Input: part model. Units: mm. Frame: model coordinates. Coordinates: 2 decimals unless noted, no trailing zeros. Loops run counter-clockwise (first coordinate to the right, second up) from the corner with the lowest first, then second, coordinate; pieces in that order, holes last. Notation, with made-up numbers: (49.5, 89.25) - (65.5, 89.25) arc R25 ccw to (65.5, 126.25) - close; hole circle Ø7 at (14, 42). An arc over 180 degrees is marked (long way). Use one line per item in the form item = value.
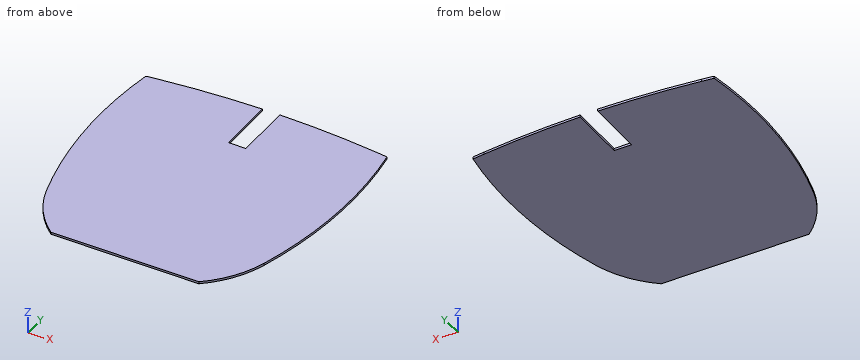
from build123d import *

# Parameters (mm, degrees)
F1_DEPTH = 0.5


with BuildPart() as f1:
    # F0 (on Top) → F1 (new body)
    with BuildSketch(Plane.XY):
        with BuildLine():
            ThreePointArc((-2, 57.790434), (-13.520553, 57.362383), (-25, 56.3))
            ThreePointArc((-25, 56.3), (-26.350558, 56.132887), (-27.7, 55.956987))
            ThreePointArc((-27.7, 55.956987), (-28.812855, 33.827216), (-25, 12))
            ThreePointArc((-25, 12), (-21.917468, 5.388354), (-17, 0))
            Line((-17, 0), (17, 0))
            ThreePointArc((17, 0), (21.917468, 5.388354), (25, 12))
            ThreePointArc((25, 12), (28.812855, 33.827216), (27.7, 55.956987))
            ThreePointArc((27.7, 55.956987), (26.350558, 56.132887), (25, 56.3))
            ThreePointArc((25, 56.3), (13.520553, 57.362383), (2, 57.790434))
            Line((2, 57.790434), (2, 44.4))
            Line((2, 44.4), (-2, 44.4))
            Line((-2, 44.4), (-2, 57.790434))
        make_face()
    extrude(amount=F1_DEPTH)


solid = f1.part
Q1. Ray query, line 1 along Y through (x, z) = (-1, 0.3); line 2 along X through (y, z) = (49, 0.15); line 3 along Y through (x, z) = (-3, 0.15). Return the intervals inside material, ascending. Write a range as [from, to].
Check values:
line_1 = [0, 44.4]
line_2 = [-28.59, -2], [2, 28.59]
line_3 = [0, 57.78]
Q2. Cut plane A-A, the plane y = 51. Return loops of the section in (x, z), then the cut area to 3 significant figures.
Check values:
outline = (-28.38, 0) - (-2, 0) - (-2, 0.5) - (-28.38, 0.5) - close; (2, 0) - (28.38, 0) - (28.38, 0.5) - (2, 0.5) - close
area = 26.4 mm²
Q3. Cut plane C-C, the plane x = -18. Return loops of the section in (y, z).
Check values:
outline = (0.85, 0) - (57.02, 0) - (57.02, 0.5) - (0.85, 0.5) - close
Q4. First-contact query: P1, Ø10, axis at x = 20.5, y = 20, coming from the -Z side. Flat tip, straight axial feed; report the tip coordinate or a pass-through.
Check values:
P1 = 0
Q5. Cut plane D-D, the plane y = 4. Return loops of the section in (x, z), then the cut area to 3 significant figures.
Check values:
outline = (-20.92, 0) - (20.92, 0) - (20.92, 0.5) - (-20.92, 0.5) - close
area = 20.9 mm²
Q6. Cut plane B-B, the plane z = 0.3. Return loops of the section in (x, y).
Check values:
outline = (-27.7, 55.96) arc R99.49 ccw to (-25, 12) arc R24.13 ccw to (-17, 0) - (17, 0) arc R24.13 ccw to (25, 12) arc R99.49 ccw to (27.7, 55.96) arc R209.08 ccw to (25, 56.3) arc R209.08 ccw to (2, 57.79) - (2, 44.4) - (-2, 44.4) - (-2, 57.79) arc R209.08 ccw to (-25, 56.3) arc R209.08 ccw to start
